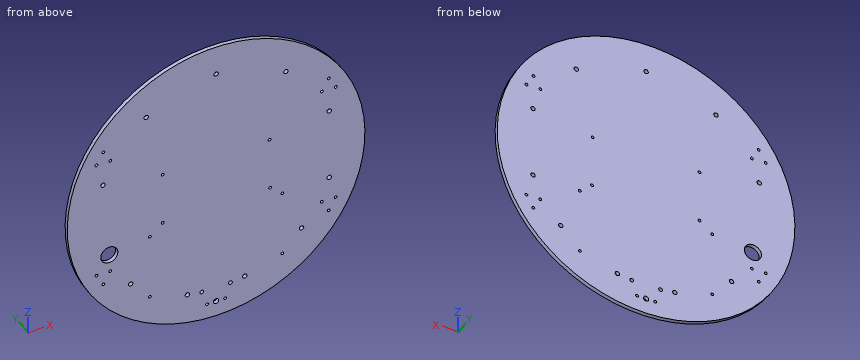
```python
from build123d import *

# Parameters (mm, degrees)
SKETCH1_R         = 177
PLATE_DEPTH       = 4.7625
SKETCH2_R         = 1.7
STANDOFFS_DEPTH   = 251.361102023
SKETCH3_R         = 1.7
LIDAR_DEPTH       = 251.361102023
SKETCH4_R         = 2.286
CAMERA_DEPTH      = 251.361102023
SKETCH5_R         = 1.7
DISPLAY_DEPTH     = 251.361102023
SKETCH6_R         = 10.16
WIRES_2_DEPTH     = 251.361102023
SKETCH7_R         = 3.175
SKETCH7_R_2       = 1.7
ARDUCAM_DEPTH     = 251.361102023
ZIPTIE_DEPTH      = 251.361102023
ZIPTIE_DEPTH_BACK = 251.361102023
SKETCH8_R         = 2.667


with BuildPart() as part:
    # Sketch1 → Plate (new body)
    with BuildSketch(Plane(origin=(0, 0, 0), x_dir=(1, 0, 0), z_dir=(0, 1, 0))):
        with Locations(Location((0, 0, 0), (0, 0, 90))):
            Circle(SKETCH1_R)
    extrude(amount=PLATE_DEPTH)

    # Sketch2 → Standoffs (cut, through all)
    with BuildSketch(Plane(origin=(0, 4.7625, 0), x_dir=(1, 0, 0), z_dir=(0, 1, 0))):
        with Locations(Location((134.039081871, -86.9125, 0), (0, 0, 270))):
            Circle(SKETCH2_R)
        with Locations(Location((125.7901899, -72.625, 0), (0, 0, 270))):
            Circle(SKETCH2_R)
        with Locations(Location((142.287973842, -72.625, 0), (0, 0, 270))):
            Circle(SKETCH2_R)
        with Locations(Location((-142.287973842, -72.625, 0), (0, 0, 270))):
            Circle(SKETCH2_R)
        with Locations(Location((-125.7901899, -72.625, 0), (0, 0, 270))):
            Circle(SKETCH2_R)
        with Locations(Location((-134.039081871, -86.9125, 0), (0, 0, 270))):
            Circle(SKETCH2_R)
        with Locations(Location((-134.039081871, 86.9125, 0), (0, 0, 270))):
            Circle(SKETCH2_R)
        with Locations(Location((-125.7901899, 72.625, 0), (0, 0, 270))):
            Circle(SKETCH2_R)
        with Locations(Location((-142.287973842, 72.625, 0), (0, 0, 270))):
            Circle(SKETCH2_R)
        with Locations(Location((142.287973842, 72.625, 0), (0, 0, 270))):
            Circle(SKETCH2_R)
        with Locations(Location((125.7901899, 72.625, 0), (0, 0, 270))):
            Circle(SKETCH2_R)
        with Locations(Location((134.039081871, 86.9125, 0), (0, 0, 270))):
            Circle(SKETCH2_R)
    extrude(amount=-STANDOFFS_DEPTH, mode=Mode.SUBTRACT)

    # Sketch3 → LIDAR (cut, through all)
    with BuildSketch(Plane(origin=(0, 4.7625, 0), x_dir=(1, 0, 0), z_dir=(0, 1, 0))):
        with Locations(Location((64.276474969, 31.75, 0), (0, 0, 270))):
            Circle(SKETCH3_R)
        with Locations(Location((-63.5, 31.75, 0), (0, 0, 270))):
            Circle(SKETCH3_R)
        with Locations(Location((-63.5, -31.75, 0), (0, 0, 270))):
            Circle(SKETCH3_R)
        with Locations(Location((63.5, -31.745252473, 0), (0, 0, 270))):
            Circle(SKETCH3_R)
    extrude(amount=-LIDAR_DEPTH, mode=Mode.SUBTRACT)

    # Sketch4 → Camera (cut, through all)
    with BuildSketch(Plane(origin=(0, 4.7625, 0), x_dir=(1, 0, 0), z_dir=(0, 1, 0))):
        with Locations(Location((-17.145, 139.7, 0), (0, 0, 270))):
            Circle(SKETCH4_R)
        with Locations(Location((17.145, 139.7, 0), (0, 0, 270))):
            Circle(SKETCH4_R)
    extrude(amount=-CAMERA_DEPTH, mode=Mode.SUBTRACT)

    # Sketch5 → Display (cut, through all)
    with BuildSketch(Plane(origin=(0, 4.7625, 0), x_dir=(1, 0, 0), z_dir=(0, 1, 0))):
        with Locations(Location((78.74500001, 123.61, 0), (0, 0, 270))):
            Circle(SKETCH5_R)
        with Locations(Location((-78.74499999, 123.61, 0), (0, 0, 270))):
            Circle(SKETCH5_R)
        with Locations(Location((78.74500001, 44.45, 0), (0, 0, 270))):
            Circle(SKETCH5_R)
        with Locations(Location((-78.74499999, 44.45, 0), (0, 0, 270))):
            Circle(SKETCH5_R)
    extrude(amount=-DISPLAY_DEPTH, mode=Mode.SUBTRACT)

    # Sketch6 → Wires 2 (cut, through all)
    with BuildSketch(Plane(origin=(0, 4.7625, 0), x_dir=(1, 0, 0), z_dir=(0, 1, 0))):
        with Locations(Location((-127, 50.8, 0), (0, 0, 270))):
            Circle(SKETCH6_R)
    extrude(amount=-WIRES_2_DEPTH, mode=Mode.SUBTRACT)

    # Sketch7 → Arducam (cut, through all)
    with BuildSketch(Plane(origin=(0, 4.7625, 0), x_dir=(1, 0, 0), z_dir=(0, 1, 0))):
        with Locations(Location((0, 157.95, 0), (0, 0, 270))):
            Circle(SKETCH7_R)
        with Locations(Location((-10.795, 157.95, 0), (0, 0, 270))):
            Circle(SKETCH7_R_2)
        with Locations(Location((10.795, 157.95, 0), (0, 0, 270))):
            Circle(SKETCH7_R_2)
    extrude(amount=-ARDUCAM_DEPTH, mode=Mode.SUBTRACT)

    # Sketch8 → Ziptie (cut, two sides: drawn at the far end of the back side and taken through both)
    with BuildSketch(Plane(origin=(0, 4.7625, 0), x_dir=(1, 0, 0), z_dir=(0, 1, 0)).offset(-ZIPTIE_DEPTH_BACK)):
        with Locations(Location((0, -141.439999949, 0), (0, 0, 270))):
            Circle(SKETCH8_R)
        with Locations(Location((-83.136346054, -114.427363643, 0), (0, 0, 270))):
            Circle(SKETCH8_R)
        with Locations(Location((-134.517433616, -43.707363669, 0), (0, 0, 270))):
            Circle(SKETCH8_R)
        with Locations(Location((134.517433616, 43.707363669, 0), (0, 0, 270))):
            Circle(SKETCH8_R)
        with Locations(Location((134.517433616, -43.707363669, 0), (0, 0, 270))):
            Circle(SKETCH8_R)
        with Locations(Location((83.136346054, -114.427363643, 0), (0, 0, 270))):
            Circle(SKETCH8_R)
        with Locations(Location((-101.628042455, 98.371818051, 0), (0, 0, 270))):
            Circle(SKETCH8_R)
        with Locations(Location((-34.100478647, 137.267734578, 0), (0, 0, 270))):
            Circle(SKETCH8_R)
        with Locations(Location((101.628042455, 98.371818051, 0), (0, 0, 270))):
            Circle(SKETCH8_R)
        with Locations(Location((34.100478647, 137.267734578, 0), (0, 0, 270))):
            Circle(SKETCH8_R)
    extrude(amount=ZIPTIE_DEPTH + ZIPTIE_DEPTH_BACK, mode=Mode.SUBTRACT)


solid = part.part
```
Model file for the job. Use its own axes, mm. Give positions to 0.01 mm unless a question says otherwise; leave off trailing zeros. Loops run counter-clockwise (first coordinate to the right, second up) from the corner with the lowest first, then second, coordinate; pieces in that order, holes last. Notation, with made-up numbers: (76, 60) -> (99, 60) arc R22 cw to (99, 77) -> close; hole circle Ø3 at (10.25, 5.25). An arc over 180 degrees is marked (long way). Use CSV: the item, a comma, the result in double quotes. Start each with the question number.
1) Slice it at D-D on z = -130. Give the cut face in (x, y).
2) Slice it at C-C on x = -153.5. Give the cut face in (y, z), plus the area to 3 significant figures.
3) Slice it at B-B on y = 3.35. Give the number of separate pieces and of enclosed holes in the cut face, plus the area to 3 significant figures.
4) Slice it at A-A on z = -56. Give the cut face in (x, y).
5) Wall check: line 1 (X direction, y = 1.9, z = -157.95) (3 decimals); line 2 (Z direction, x = -5, y = 3.2); line 3 (X direction, y = 3.5, z = -139.7). Give the ranges that are in metal, low to high.
6) Flat gauge pins, fed straight in: pin 1 Ø1 at (x, y) = (-90, 2) entering from +Z; pin 2 Ø2 at (x, y) = (-38.5, 3) entering from +Z. Where does each tip first touch, or does it go through?
Computed values:
1,outline,"(-120.12, 0) -> (120.12, 0) -> (120.12, 4.76) -> (-120.12, 4.76) -> close"
2,outline,"(0, -88.13) -> (4.76, -88.13) -> (4.76, 88.13) -> (0, 88.13) -> close"
2,area,"839 mm^2"
3,separate pieces,"1"
3,enclosed holes,"36"
3,area,"97,600 mm^2"
4,outline,"(-167.91, 0) -> (-135.73, 0) -> (-135.73, 4.76) -> (-167.91, 4.76) -> close; (-118.27, 0) -> (167.91, 0) -> (167.91, 4.76) -> (-118.27, 4.76) -> close"
5,line 1,"x = -79.88 to -12.495, -9.095 to -3.175, 3.175 to 9.095, 12.495 to 79.88"
5,line 2,"z = -176.93 to 176.93"
5,line 3,"x = -108.69 to -35.19, -33.01 to -19.43, -14.86 to 14.86, 19.43 to 33.01, 35.19 to 108.69"
6,pin 1,"stops at z = 152.7"
6,pin 2,"stops at z = 172.98"
